Check sheet for the drawn part. Datum: minimum x, y, z corner. Units: mm. A direction names the side the tool comes from. Give positions to 0.01 mm unless a question says otherwise; leave off trailing zeros. Order: outer loops, then holes, each group sorted by start corner. A loop starts at its lowest first (then second) coordinate and runs counter-clockwise, first axis right, second up. Notation, with made-up numbers: (72, -37.5) -> (118, -37.5) arc R10 cw to (118, -26.5) -> close; hole circle Ø10 at (-17.5, 3.5). An arc over 180 degrees is marked (long way). One line per question, with ' | ' between items. Start each with the question number.
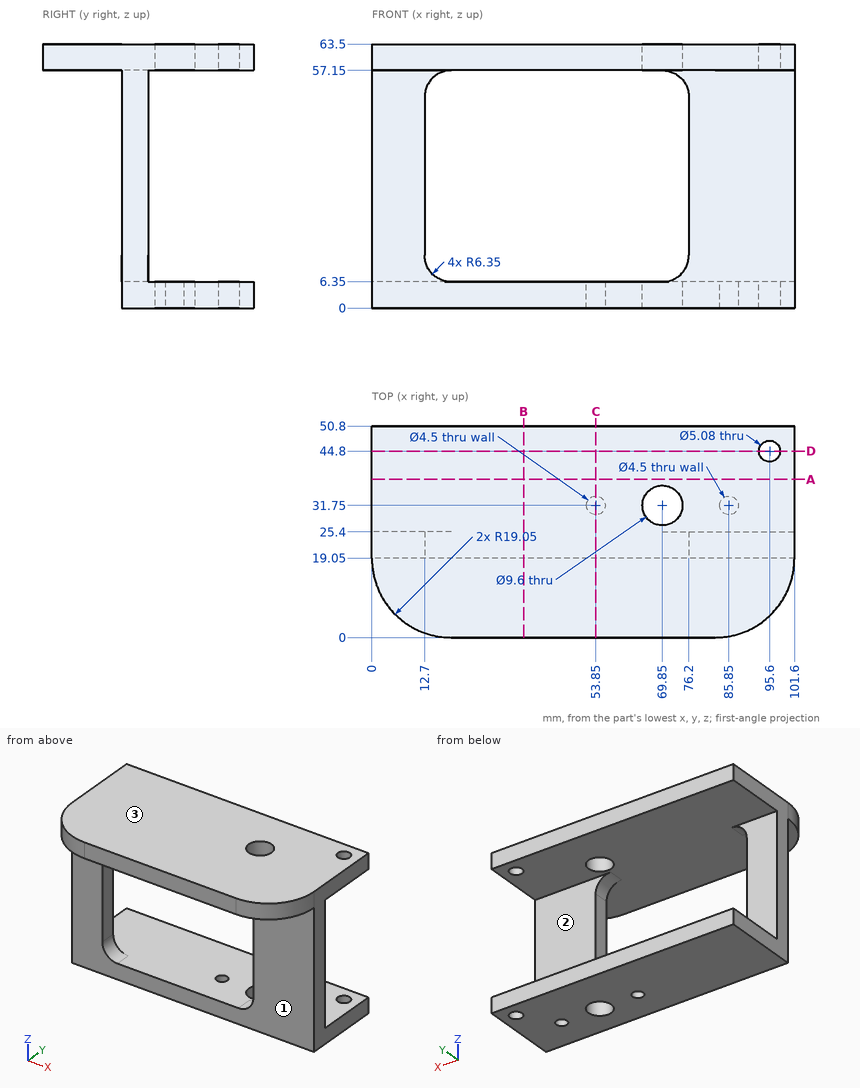
1. Cross-section at A-A on y = 38. Record the boundary of the cut face in (x, z), and give its area (3 significant figures).
2. Cross-section at D-D on y = 44.8. Record the boundary of the cut face in (x, z), and give its area (3 significant figures).
3. Cross-section at C-C on x = 53.85. Record the boundary of the cut face in (y, z).
4. Tool access check on the marked faces 1, 2 and 3. Record the directions out of +Z, -Z, +X, -X, +Y, -Y that give a thin tool (end or side, any length) a straight path to the whole face; none if there is none.
5. Scan lines: probe 1 along Z at (x, y) = (58, 48); probe 2 along X at (y, z) = (31, 2); probe 3 along Y at (x, z) = (95.6, 2.75). Record each from-to range of solid material in increasing order.
6. Go/stop test with flat-tipped pins: pin 1 (1 mm diameter, centred on x = 62.5, y = 15, fed in from -Z); pin 2 (9.5 mm diameter, centred on x = 88, z = 22, fed in from +Y). Record where each tip stops, or that it passes through.
7. Cross-section at B-B on x = 36.5. Record the boundary of the cut face in (y, z), and give its area (3 significant figures).
Response values:
1) outline: (0, 0) -> (101.6, 0) -> (101.6, 6.35) -> (0, 6.35) -> close; (0, 57.15) -> (101.6, 57.15) -> (101.6, 63.5) -> (0, 63.5) -> close | area: 1,290 mm²
2) outline: (0, 0) -> (93.06, 0) -> (93.06, 6.35) -> (0, 6.35) -> close; (0, 57.15) -> (93.06, 57.15) -> (93.06, 63.5) -> (0, 63.5) -> close; (98.14, 0) -> (101.6, 0) -> (101.6, 6.35) -> (98.14, 6.35) -> close; (98.14, 57.15) -> (101.6, 57.15) -> (101.6, 63.5) -> (98.14, 63.5) -> close | area: 1,230 mm²
3) outline: (0, 57.15) -> (50.8, 57.15) -> (50.8, 63.5) -> (0, 63.5) -> close; (19.05, 0) -> (29.5, 0) -> (29.5, 6.35) -> (19.05, 6.35) -> close; (34, 0) -> (50.8, 0) -> (50.8, 6.35) -> (34, 6.35) -> close
4) face 1: -Z, +X, -X, -Y | face 2: +X, -X, +Y | face 3: +Z, +X, -X, +Y, -Y
5) probe 1: z = 0 to 6.35, 57.15 to 63.5 | probe 2: x = 0 to 51.73, 55.97 to 65.11, 74.59 to 83.73, 87.97 to 101.6 | probe 3: y = 19.05 to 42.26, 47.34 to 50.8
6) pin 1: stops at z = 57.15 | pin 2: stops at y = 25.4
7) outline: (0, 57.15) -> (50.8, 57.15) -> (50.8, 63.5) -> (0, 63.5) -> close; (19.05, 0) -> (50.8, 0) -> (50.8, 6.35) -> (19.05, 6.35) -> close | area: 524 mm²
